from build123d import *

# Parameters (mm, degrees)
LEFT_CROSS_SECTION_SKETCH_R   = 15
RIGHT_START                   = 100
RIGHT_CROSS_SECTION_SKETCH_R  = 15
RIGHT_JOINT_EXTRUDE_DEPTH     = 100
LEFT_CROSS_SECTION_SKETCH_2_R = 15
LEFT_JOINT_EXTRUDE_DEPTH      = 100


with BuildPart() as part:
    # Bar Sweep: sweep along a path in Overhead Sketch
    with BuildLine(Plane(origin=(0, 0, 0), x_dir=(1, 0, 0), z_dir=(0, 1, 0))) as bar_sweep_path:
        Line((517.079999105, -433.881636538), (539.572146309, -452.754788961))
        ThreePointArc((539.572146309, -452.754788961), (550.223234493, -473.758055128), (542.428454955, -495.980212564))
        ThreePointArc((542.428454955, -495.980212564), (0, -735), (-542.428454955, -495.980212564))
        ThreePointArc((-542.428454955, -495.980212564), (-550.223234493, -473.758055128), (-539.572146309, -452.754788961))
        Line((-539.572146309, -452.754788961), (-517.079999105, -433.881636538))
    # Left Cross Section Sketch → Bar Sweep (sweep)
    with BuildSketch(Plane(origin=(517.079999105, 0, 433.881636538), x_dir=(0.6427876096865377, 0, -0.7660444431189796), z_dir=(0.7660444431189796, 0, 0.6427876096865377))):
        Circle(LEFT_CROSS_SECTION_SKETCH_R)
    sweep(path=bar_sweep_path.line)

    # Right Cross Section Sketch → Right Joint Extrude (add)
    with BuildSketch(Plane(origin=(-517.079999105, 0, 433.881636538), x_dir=(-0.642787609686537, 0, -0.7660444431189801), z_dir=(0.7660444431189801, 0, -0.6427876096865369)).offset(RIGHT_START)):
        Circle(RIGHT_CROSS_SECTION_SKETCH_R)
    extrude(amount=-RIGHT_JOINT_EXTRUDE_DEPTH)

    # Left Cross Section Sketch<2> → Left Joint Extrude (add)
    with BuildSketch(Plane(origin=(517.079999105, 0, 433.881636538), x_dir=(0.6427876096865377, 0, -0.7660444431189796), z_dir=(0.7660444431189796, 0, 0.6427876096865377))):
        Circle(LEFT_CROSS_SECTION_SKETCH_2_R)
    extrude(amount=-LEFT_JOINT_EXTRUDE_DEPTH)


solid = part.part
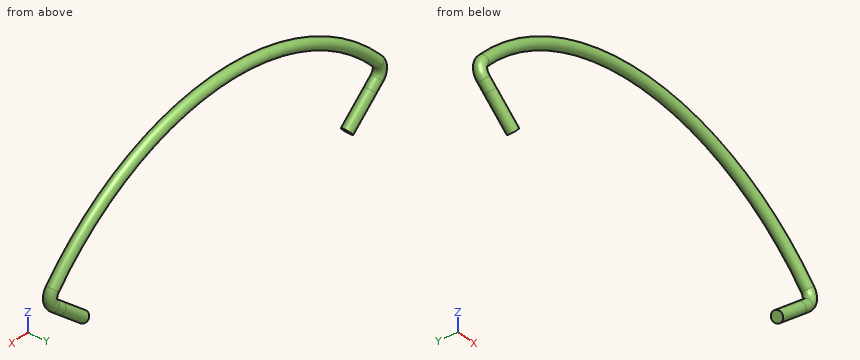
The model under review builds one solid part; all positions refer to its coordinate system, in mm. Round coordinates to 2 decimals unless told otherwise and drop trailing zeros. Order: outer loops, then holes, each group sorted by start corner. A loop starts at its lowest first (then second) coordinate and runs counter-clockwise, first axis right, second up. Notation, with made-up numbers: (46.25, 21.5) - (105.25, 21.5) arc R20 cw to (105.25, 55.5) - close; hole circle Ø2 at (6, 13). An arc over 180 degrees is marked (long way). Use one line per item in the form item = value.
Q1. To check wall thickness, follow line 1 (X direction, y = 2, z = 631.5); line 2 (X direction, y = -8, z = 527.5); line 3 (Z direction, x = -455, y = 7). State the ranges of each line that lie inside material, in increasing order.
Response values:
line_1 = -404.36 to -346.12, 346.12 to 404.36
line_2 = -529.89 to -493.43, 493.43 to 529.89
line_3 = 364.47 to 399.11, 560.24 to 594.04
Q2. Clearance check with flat-ended pins moving along their axes: P1, Ø2, axis at y = -8, z = 657.5, coming from the +X side; P2, Ø4, axis at x = -45.5, y = 5.5, coming from the -Z side; P3, Ø1.5, axis at x = -247.5, y = 4.5, coming from the +Z side. State where each tip first meets the part, or that it passes through.
Response values:
P1 = 358.22
P2 = 718.96
P3 = 707.61
Q3. Add section A-A on y = -7.5. Give the boundary of the cut face in (x, z), then the cut area to 3 significant figures.
Response values:
outline = (-552.02, 504.75) arc R42.99 ccw to (-547.92, 442.8) - (-448.83, 359.65) - (-432.13, 379.55) - (-531.22, 462.71) arc R17.01 cw to (-532.84, 487.21) arc R722.01 cw to (532.84, 487.21) arc R17.01 cw to (531.22, 462.71) - (432.13, 379.55) - (448.83, 359.65) - (547.92, 442.8) arc R42.99 ccw to (552.02, 504.75) arc R747.99 ccw to start
area = 40,900 mm^2
